from build123d import *

# Parameters (mm, degrees)
F0_W     = 150
F0_H     = 90
F0_R     = 25
F1_DEPTH = 45
F2_W     = 6.35
F2_H     = 90
F3_DEPTH = 12.7


# Not quite as in the source:
# - a feature names something its author has since deleted; it is built from what else it names


with BuildPart() as f1:
    # F0 (on Top) → F1 (new body)
    with BuildSketch(Plane.XY):
        Rectangle(F0_W, F0_H)
        Circle(F0_R, mode=Mode.SUBTRACT)
    extrude(amount=F1_DEPTH)

    # F2 (on face) → F3 (cut)
    with BuildSketch(Plane.XY.offset(45)):
        with Locations((-69.285, 0)):
            Rectangle(F2_W, F2_H)
        with BuildLine():
            Line((-9.525, -23.1143759379), (-9.525, -45))
            Line((-9.525, -45), (9.525, -45))
            Line((9.525, -45), (9.525, -23.1143759379))
            ThreePointArc((9.525, -23.1143759379), (0, -25), (-9.525, -23.1143759379))
        make_face()
        with BuildLine():
            Line((9.525, 45), (-9.525, 45))
            Line((-9.525, 45), (-9.525, 23.1143759379))
            ThreePointArc((-9.525, 23.1143759379), (0, 25), (9.525, 23.1143759379))
            Line((9.525, 23.1143759379), (9.525, 45))
        make_face()
    extrude(amount=-F3_DEPTH, mode=Mode.SUBTRACT)


solid = f1.part
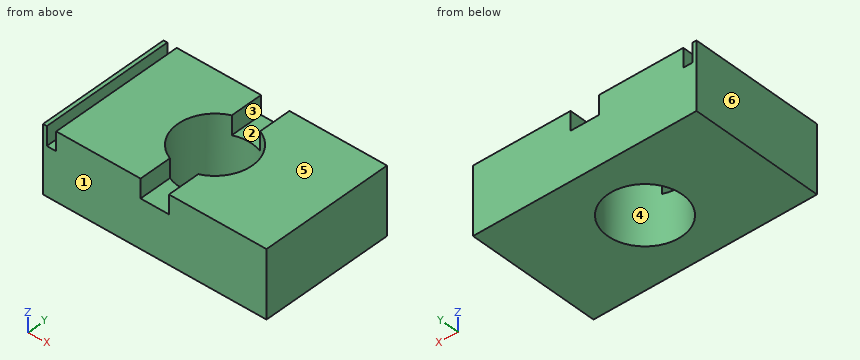
Geometry: final body of the model. Coordinates: model frame, mm. Face numbers are marked on the shaded views. A direction names the side the tool comes from. Give positions to 0.01 mm unless a question says otherwise; leave off trailing zeros. Order: outer loops, then holes, each group sorted by start corner. A loop starts at its lowest first (then second) coordinate and runs counter-clockwise, first axis right, second up. Notation, with made-up numbers: (16, 29) -> (41, 29) arc R29 ccw to (41, 63) -> close; hole circle Ø1 at (77, 59.5). An arc over 180 degrees is marked (long way). Put each result on its own line as item: value.
Q1. Section D-D, the plane y = 37. Return loops of the section in (x, z) (3 decimals), then the cut area to 3 significant figures.
Here are the results:
outline: (-75, 0) -> (75, 0) -> (75, 45) -> (9.525, 45) -> (9.525, 32.3) -> (-9.525, 32.3) -> (-9.525, 45) -> (-66.11, 45) -> (-66.11, 32.3) -> (-72.46, 32.3) -> (-72.46, 45) -> (-75, 45) -> close
area: 6,430 mm^2
Q2. Draft query along X for the marked faces 3, 4, 5 and 6. Return one class per face: released by +X, released by -X, zero draft, split by the parting line, or undercut.
Here are the results:
face 3: undercut
face 4: undercut
face 5: zero draft
face 6: released by -X
Q3. Material intervals for L1, parallel to X at y = -31, z = 33.5 (3 decimals); L2, parallel to X at y = 0, z = 33; L3, parallel to X at y = 0, z = 21, sorted ascending.
Here are the results:
L1: x = -75 to -72.46, -66.11 to -9.525, 9.525 to 75
L2: x = -75 to -72.46, -66.11 to -25, 25 to 75
L3: x = -75 to -25, 25 to 75
Q4. Section B-B, the plane y = -15. Return loops of the section in (x, z).
Here are the results:
outline: (-75, 0) -> (-20, 0) -> (-20, 45) -> (-66.11, 45) -> (-66.11, 32.3) -> (-72.46, 32.3) -> (-72.46, 45) -> (-75, 45) -> close; (20, 0) -> (75, 0) -> (75, 45) -> (20, 45) -> close
Q5. Reachability of the marked faces 1 and 2 from +Z, -Z, +X, -X, +Y, -Y: full face, straight path, thin tool, end or side. Return the list, or none.
Here are the results:
face 1: +Z, -Z, +X, -X, -Y
face 2: +Z, +Y, -Y
Q6. Section C-C, the plane z = 4. Return loops of the section in (x, y).
Here are the results:
outline: (-75, -45) -> (75, -45) -> (75, 45) -> (-75, 45) -> close; hole circle Ø50 at (0, 0)
Q7. Section A-A, the plane x = 0. Return loops of the section in (y, z).
Here are the results:
outline: (-45, 0) -> (-25, 0) -> (-25, 32.3) -> (-45, 32.3) -> close; (25, 0) -> (45, 0) -> (45, 32.3) -> (25, 32.3) -> close
Q8. Pin query (flat end, axial travel): pin 1 (9.5 mm diameter, centred on x = 2.5, y = -38, fed in from +Z). Return the tip coordinate at first contact, or that it passes through.
Here are the results:
pin 1: stops at z = 32.3
